```python
from build123d import *

# Parameters (mm, degrees)
SKETCH_W     = 28
SKETCH_H     = 13
SKETCH_R     = 1.6
PAD_DEPTH    = 3
SKETCH001_W  = 28
SKETCH001_H  = 3
PAD001_DEPTH = 13
SKETCH002_R  = 1.6
POCKET_DEPTH = 3.001
FILLET_R     = 1


with BuildPart() as part:
    # Sketch → Pad (new body)
    with BuildSketch(Plane.XY):
        with Locations((10.5, -1.5)):
            Rectangle(SKETCH_W, SKETCH_H)
        Circle(SKETCH_R, mode=Mode.SUBTRACT)
        with Locations((21, 0)):
            Circle(SKETCH_R, mode=Mode.SUBTRACT)
    extrude(amount=PAD_DEPTH)

    # Sketch001 (on Face8 of Pad) → Pad001 (join)
    with BuildSketch(Plane.XY.offset(3)):
        with Locations((10.5, -6.5)):
            Rectangle(SKETCH001_W, SKETCH001_H)
    extrude(amount=PAD001_DEPTH)

    # Sketch002 (on Face11 of Pad001) → Pocket (cut, through all)
    with BuildSketch(Plane(origin=(0, -5, 0), x_dir=(-1, 0, 0), z_dir=(0, 1, 0))):
        with Locations((-21, 8)):
            Circle(SKETCH002_R)
        with Locations((-17.5, 12)):
            Circle(SKETCH002_R)
        with Locations((-14, 8)):
            Circle(SKETCH002_R)
        with Locations((-10.5, 12)):
            Circle(SKETCH002_R)
        with Locations((-7, 8)):
            Circle(SKETCH002_R)
        with Locations((-3.5, 12)):
            Circle(SKETCH002_R)
        with Locations((0, 8)):
            Circle(SKETCH002_R)
    extrude(amount=-POCKET_DEPTH, mode=Mode.SUBTRACT)

    # Fillet
    fillet_edges = [part.edges().sort_by_distance(p)[0] for p in [
        (24.5, -6.5, 16),
        (-3.5, -6.5, 16),
        (-3.5, 5, 1.5),
        (24.5, 5, 1.5),
    ]]
    fillet(fillet_edges, radius=FILLET_R)


solid = part.part
```
Verification items for the finished model (mm, model axes). A direction names the side the tool comes from. Coordinates: 2 decimals unless noted, no trailing zeros. Loops run counter-clockwise (first coordinate to the right, second up) from the corner with the lowest first, then second, coordinate; pieces in that order, holes last. Notation, with made-up numbers: (19, 28) - (39, 28) arc R16 ccw to (39, 58) - close; hole circle Ø5 at (-3, 73). An arc over 180 degrees is marked (long way). Answer as a JSON object with one key per item and string values.
(1) Access from +Z, -Z, +X, -X, +Y, -Y to the whole of each face (thin tool, end or side, straight path). Record for faces 4 (the cylindrical face through (-3.215, -6.479, 15.699)), 5 (the flat face through (10, 0, 3)).
Response:
{"face 4": "+Z, -X, +Y, -Y", "face 5": "+Z, +X, -X, +Y"}
(2) Cross-section at D-D, the plane z = 12. Record the boundary of the cut face in (x, y).
Response:
{"outline": "(-3.5, -8) - (1.9, -8) - (1.9, -5) - (-3.5, -5) - close; (5.1, -8) - (8.9, -8) - (8.9, -5) - (5.1, -5) - close; (12.1, -8) - (15.9, -8) - (15.9, -5) - (12.1, -5) - close; (19.1, -8) - (24.5, -8) - (24.5, -5) - (19.1, -5) - close"}
(3) Mould release check, pull along X, two halves, no side actions. Record for faces 1 (the cylindrical face through (12.1, -6.48, 12.07)), 2 (the flat face through (10, 5, 1)), 3 (the cylindrical face through (24.199, -6.479, 15.715)): pulls with the +X half, pulls with the -X half, needs draft (parallel to the pull), parting line crosses it, or undercut.
Response:
{"face 1": "undercut", "face 2": "needs draft", "face 3": "pulls with the +X half"}
(4) Cross-section at C-C, the plane y = 0. Record the boundary of the cut face in (x, z), then the cut area to 3 significant figures.
Response:
{"outline": "(-3.5, 0) - (-1.6, 0) - (-1.6, 3) - (-3.5, 3) - close; (1.6, 0) - (19.4, 0) - (19.4, 3) - (1.6, 3) - close; (22.6, 0) - (24.5, 0) - (24.5, 3) - (22.6, 3) - close", "area": "64.8 mm²"}
(5) Go/stop test with flat-tipped pins: pin 1 Ø6 at (x, z) = (2, 7.5) entering from +Y; pin 2 Ø5 at (x, y) = (6.5, 0) entering from +Z; pin 3 Ø3 at (x, z) = (0, 8) entering from -Y. Record where each tip stops, or that it passes through.
Response:
{"pin 1": "stops at y = -5", "pin 2": "stops at z = 3", "pin 3": "passes through"}
(6) Cross-section at A-A, the plane x = 7. Record the boundary of the cut face in (y, z), then the cut area to 3 significant figures.
Response:
{"outline": "(-8, 0) - (5, 0) - (5, 3) - (-5, 3) - (-5, 6.4) - (-8, 6.4) - close; (-8, 9.6) - (-5, 9.6) - (-5, 16) - (-8, 16) - close", "area": "68.4 mm²"}
(7) Scan lines: line 1 along Z through (x, y) = (17.5, -6.4); line 2 along Z through (x, y) = (14, -7); line 3 along Y through (x, z) = (19.75, 5.75). Record each from-to range of solid material in increasing order.
Response:
{"line 1": "z = 0 to 10.4, 13.6 to 16", "line 2": "z = 0 to 6.4, 9.6 to 16", "line 3": "y = -8 to -5"}
(8) Cross-section at B-B, the plane z = 8. Record the boundary of the cut face in (x, y).
Response:
{"outline": "(-3.5, -8) - (-1.6, -8) - (-1.6, -5) - (-3.5, -5) - close; (1.6, -8) - (5.4, -8) - (5.4, -5) - (1.6, -5) - close; (8.6, -8) - (12.4, -8) - (12.4, -5) - (8.6, -5) - close; (15.6, -8) - (19.4, -8) - (19.4, -5) - (15.6, -5) - close; (22.6, -8) - (24.5, -8) - (24.5, -5) - (22.6, -5) - close"}
